Geometry check sheet. Reference: the model listing, model coordinates, mm. A direction names the side the tool comes from. Coordinates: 2 decimals unless noted, no trailing zeros. Write each loop counter-clockwise with the first axis right and the second up, starting at its lowest first coordinate (ties: lowest second). Pieces come first, ordered by that corner, then holes. Notation, with made-up numbers: (0.25, 31.5) -> (48.25, 31.5) arc R28 cw to (48.25, 60.5) -> close; hole circle Ø5 at (-7.5, 32.5). An arc over 180 degrees is marked (long way). Answer in a Markdown table with one row per item. Add a question column.
1. Cross-section at C-C on x = 1.5. Record the cut outline in (y, z), and give its area (3 significant figures).
2. Scan lines: L1, parallel to X at y = 19.75, z = 6; L2, parallel to Z at x = 3, y = 18.5; L3, parallel to X at y = 18, z = 22. Record each from-to range of solid material in increasing order. Write a range as from..to.
3. Cross-section at D-D on z = -9. Record the cut outline in (x, y).
4. Set-up check for faces 1 (the flat face through (-1.524, 14, 21)), 2 (the cylindrical face through (10.45, 3.22, 13.59)), 3 (the flat face through (-9.474, 16, 0)): record each of +Z, -Z, +X, -X, +Y, -Y from which the full face is reachable in a straight line by a thin tool's end or side.
5. Cross-section at B-B on y = 10.5. Record the cut outline in (x, z).
6. Mould release check, pull along Z, two halves, no side actions. Record for faces 4 (the cylindrical face through (16.8, 14.46, 26.29)), 5 (the flat face through (11.176, 3, 0)), 6 (the flat face through (0, 16, -7.938)): pulls with the +Z half, pulls with the -Z half, needs draft (parallel to the pull), parting line crosses it, or undercut.
7. Cross-section at A-A on z = 22. Record the cut outline in (x, y).
8. Depth check by flat-ended pin: P1, Ø2, axis at x = -5.5, z = -3, coming from the +Y side; P2, Ø1, axis at x = 7.5, z = 22.5, coming from the -Y side; P3, Ø3, axis at y = 4, z = 5.5, coming from the +X side. Enter the tip coordinate at first touch or a pass-through.
```python
from build123d import *

# Parameters (mm, degrees)
SKETCH1_W           = 35.052
SKETCH1_H           = 28.702
BOSS_EXTRUDE5_DEPTH = 22.352
SKETCH6_W           = 28.702
SKETCH6_H           = 6.35
CUT_EXTRUDE1_DEPTH  = 6.35
SKETCH7_W           = 19.05
SKETCH7_H           = 16.002
BOSS_EXTRUDE6_DEPTH = 12.7
CUT_EXTRUDE2_DEPTH  = 12.7
FILLET5_R           = 2.54
FILLET6_R           = 2.54


with BuildPart() as part:
    # Sketch1 → Boss-Extrude5 (new body)
    with BuildSketch(Plane(origin=(0, 0, 0), x_dir=(1, 0, 0), z_dir=(0, 1, 0))):
        Rectangle(SKETCH1_W, SKETCH1_H)
    extrude(amount=BOSS_EXTRUDE5_DEPTH)

    # Sketch6 → Cut-Extrude1 (cut)
    with BuildSketch(Plane(origin=(17.526, 0, 0), x_dir=(0, 0, -1), z_dir=(1, 0, 0))):
        with Locations((0, 3.175)):
            Rectangle(SKETCH6_W, SKETCH6_H)
    extrude(amount=-CUT_EXTRUDE1_DEPTH, mode=Mode.SUBTRACT)

    # Sketch7 → Boss-Extrude6 (add)
    with BuildSketch(Plane.XY.offset(14.351)):
        with Locations((8.001, 14.351)):
            Rectangle(SKETCH7_W, SKETCH7_H)
    extrude(amount=BOSS_EXTRUDE6_DEPTH)

    # Sketch8 → Cut-Extrude2 (cut)
    with BuildSketch(Plane(origin=(0, 22.352, 0), x_dir=(1, 0, 0), z_dir=(0, 1, 0))):
        Polygon((-9.4742, 7.9375), (-9.4742, -7.9375), (6.4008, -7.9375), (6.4008, -27.051), (9.5758, -27.051), (9.5758, 7.9375), align=None)
    extrude(amount=-CUT_EXTRUDE2_DEPTH, mode=Mode.SUBTRACT)

    # Fillet5
    fillet5_edges = [part.edges().sort_by_distance(p)[0] for p in [
        (11.176, 3.175, -14.351),
        (-1.524, 14.351, 14.351),
        (-17.526, 11.176, 14.351),
        (-17.526, 11.176, -14.351),
        (17.526, 14.351, -14.351),
    ]]
    fillet(fillet5_edges, radius=FILLET5_R)

    # Fillet6
    fillet6_edges = [part.edges().sort_by_distance(p)[0] for p in [
        (11.176, 3.175, 14.351),
        (-1.524, 14.351, 27.051),
        (17.526, 14.351, 27.051),
    ]]
    fillet(fillet6_edges, radius=FILLET6_R)


solid = part.part
```
Results found:
| question | item | result |
|---|---|---|
| 1 | outline | (0, -14.35) -> (22.35, -14.35) -> (22.35, -7.94) -> (9.65, -7.94) -> (9.65, 7.94) -> (22.35, 7.94) -> (22.35, 27.05) -> (6.35, 27.05) -> (6.35, 14.35) -> (0, 14.35) -> close |
| 1 | area | 643 mm^2 |
| 2 | L1 | x = -17.53..-9.47, 9.58..17.53 |
| 2 | L2 | z = -14.35..-7.94, 7.94..27.05 |
| 2 | L3 | x = -1.52..6.4, 9.58..17.53 |
| 3 | outline | (-17.53, 0) -> (11.18, 0) -> (11.18, 6.35) -> (17.53, 6.35) -> (17.53, 22.35) -> (-17.53, 22.35) -> close |
| 4 | face 1 | +Z, -X, +Y, -Y |
| 4 | face 2 | +Z, +X, -Y |
| 4 | face 3 | +Y |
| 5 | outline | (-17.53, -11.81) arc R2.54 ccw to (-14.99, -14.35) -> (14.99, -14.35) arc R2.54 ccw to (17.53, -11.81) -> (17.53, 24.51) arc R2.54 ccw to (14.99, 27.05) -> (9.58, 27.05) -> (9.58, -7.94) -> (-9.47, -7.94) -> (-9.47, 7.94) -> (6.4, 7.94) -> (6.4, 27.05) -> (1.02, 27.05) arc R2.54 ccw to (-1.52, 24.51) -> (-1.52, 16.89) arc R2.54 cw to (-4.06, 14.35) -> (-14.99, 14.35) arc R2.54 ccw to (-17.53, 11.81) -> close |
| 6 | face 4 | pulls with the +Z half |
| 6 | face 5 | needs draft |
| 6 | face 6 | undercut |
| 7 | outline | (-1.52, 6.35) -> (17.53, 6.35) -> (17.53, 22.35) -> (9.58, 22.35) -> (9.58, 9.65) -> (6.4, 9.65) -> (6.4, 22.35) -> (-1.52, 22.35) -> close |
| 8 | P1 | stops at y = 9.65 |
| 8 | P2 | stops at y = 6.35 |
| 8 | P3 | stops at x = 11.18 |
